Solid Edge part; units mm, degrees
sketch "Sketch1" plane through (0, 0, 0) normal (1, 0, 0) x (0, 1, 0)
  circle A0 centre (0, 0) radius 20
  circle A1 centre (0, 0) radius 83.875
extrude "Protrusion1" add sketch "Sketch1" along normal mid plane 69
sketch "Sketch2" plane through (34.5, 0, 0) normal (1, 0, 0) x (0, 1, 0)
  circle A0 centre (0, 0) radius 70
  circle A1 centre (0, 0) radius 25
extrude "VaciadoExtruido_1" cut sketch "Sketch2" against normal blind 15
sketch "Sketch3" plane through (-34.5, 0, 0) normal (-1, 0, 0) x (0, -1, 0)
  circle A0 centre (0, 0) radius 70
  circle A1 centre (0, 0) radius 25
extrude "VaciadoExtruido_2" cut sketch "Sketch3" against normal blind 15
sketch "Sketch4" plane through (34.5, 0, 0) normal (1, 0, 0) x (0, 1, 0)
  line L0 (0, 23.1) -> (-6, 23.1)
  line L1 (-6, 23.1) -> (-6, 19.0788)
  line L2 (6, 23.1) -> (6, 19.0788)
  line L3 (0, 23.1) -> (6, 23.1)
  arc A0 (-6, 19.0788) -> (6, 19.0788) centre (0, 0) cw
extrude "Cutout1" cut sketch "Sketch4" along normal mid plane 368
properties material "Acero"
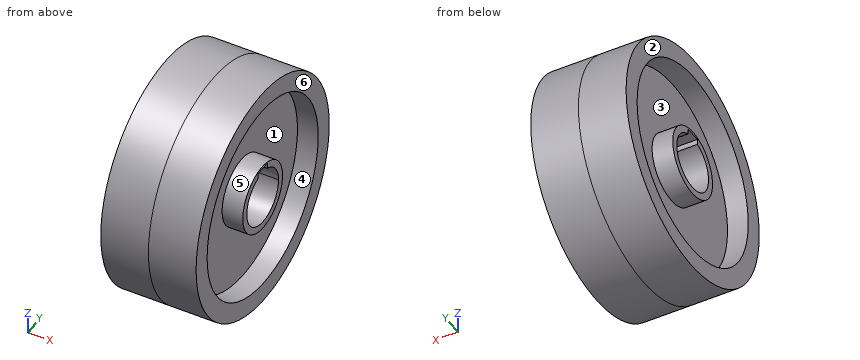
Read the model definition and answer for the solid it produces. Units are mm, in the model's axes. Face numbers are marked on the shaded views. A direction names the side the tool comes from. Round coordinates to 2 decimals unless told otherwise and drop trailing zeros. Write each loop counter-clockwise with the first axis right and the second up, starting at its lowest first coordinate (ties: lowest second). Pieces come first, ordered by that corner, then holes. Notation, with made-up numbers: (53, -20) - (74, -20) arc R31 cw to (74, 14) - close; hole circle Ø11 at (86, 83). An arc over 180 degrees is marked (long way). Use CSV: the item, a comma, the result in double quotes.
Q1. Find section C-C, the plane x = -13.5. Write down the section's boundary in (y, z) (3 decimals), then the cut area to 3 significant figures.
Values:
outline,"circle Ø167.75 at (0, 0); hole (-6, 19.079) arc R20 ccw (long way) to (6, 19.079) - (6, 23.1) - (-6, 23.1) - close"
area,"20,800 mm²"
Q2. Determine the mould class of the marked faces 4, 5 and 6 for opening direction Z: +Z half, -Z half, draft (parallel to the pull), parting line (faces both ways), or undercut.
Values:
face 4,"undercut"
face 5,"undercut"
face 6,"draft"
Q3. A tool of negligible diameter and unlimited length cuts with its end or side. For the marked faces 1, 2 and 3, from which of +Z, -Z, +X, -X, +Y, -Y can it reach the whole face along a straight path? Write none if from no direction.
Values:
face 1,"+X"
face 2,"+Z, -Z, -X, +Y, -Y"
face 3,"-X"
Q4. Each of these flat-tipped pins is pushed along its axis until it touches: pin 1 Ø2 at (y, z) = (39, 23.5) entering from -X; pin 2 Ø5 at (x, z) = (-23, -42.5) entering from -Y; pin 3 Ø1.2 at (x, z) = (6.5, 22) entering from +Y. Where does it stop, or does it pass through?
Values:
pin 1,"stops at x = -19.5"
pin 2,"stops at y = -73.72"
pin 3,"stops at y = 81.1"
Q5. Find section D-D, the plane y = 62. Write down the section's boundary in (x, z), then the cut area to 3 significant figures.
Values:
outline,"(-34.5, -56.49) - (34.5, -56.49) - (34.5, -32.5) - (19.5, -32.5) - (19.5, 32.5) - (34.5, 32.5) - (34.5, 56.49) - (-34.5, 56.49) - (-34.5, 32.5) - (-19.5, 32.5) - (-19.5, -32.5) - (-34.5, -32.5) - close"
area,"5,850 mm²"
Q6. Find section B-B, the plane y = 0. Write down the section's boundary in (x, z) (3 decimals).
Values:
outline,"(-34.5, -83.875) - (34.5, -83.875) - (34.5, -70) - (19.5, -70) - (19.5, -25) - (34.5, -25) - (34.5, -20) - (-34.5, -20) - (-34.5, -25) - (-19.5, -25) - (-19.5, -70) - (-34.5, -70) - close; (-34.5, 23.1) - (34.5, 23.1) - (34.5, 25) - (19.5, 25) - (19.5, 70) - (34.5, 70) - (34.5, 83.875) - (-34.5, 83.875) - (-34.5, 70) - (-19.5, 70) - (-19.5, 25) - (-34.5, 25) - close"
Q7. Straight lines are drawn through the part: line 1 along Z through (x, y) = (-20, 0) (3 decimals); line 2 along Z through (x, y) = (9, 0) (3 decimals); line 3 along X through (y, z) = (-25.5, 58.5). For each, find the intervals that lie inside material, in ascending order.
Values:
line 1,"z = -83.875 to -70, -25 to -20, 23.1 to 25, 70 to 83.875"
line 2,"z = -83.875 to -20, 23.1 to 83.875"
line 3,"x = -19.5 to 19.5"
Q8. Find section A-A, the plane x = -23. Write down the section's boundary in (y, z) (3 decimals), then the cut area to 3 significant figures.
Values:
outline,"circle Ø167.75 at (0, 0); circle Ø50 at (0, 0); hole circle Ø140 at (0, 0); hole (-6, 19.079) arc R20 ccw (long way) to (6, 19.079) - (6, 23.1) - (-6, 23.1) - close"
area,"7,370 mm²"
